Input: part model. Units: mm. Frame: model coordinates. Face numbers are marked on the shaded views. A direction names the side the tool comes from. Give positions to 0.01 mm unless a question says otherwise; leave off trailing zeros. Write each loop counter-clockwise with the first axis right and the second up, starting at its lowest first coordinate (ties: lowest second). Pieces come first, ordered by that corner, then holes. Notation, with made-up numbers: (-34.5, -1.75) - (-11.5, -1.75) arc R33 cw to (-11.5, 27.25) - close; hole circle Ø4 at (-27.75, 49.5). An arc over 180 degrees is marked (long way). Use a Markdown table: item, result. Add a question column.
1. Set-up query: the marked faces 1 and 2. Return all of +Z, -Z, +X, -X, +Y, -Y with unobstructed straight access to the full face (end or side cutting, diameter ignored); none if empty.
2. Section query C-C, the plane z = -82. Return loops of the section in (x, y).
3. Material intervals for probe 1 along Z at (x, y) = (-10.5, -1.5); probe 2 along X at (y, z) = (25, -56.5); probe 3 along Y at (x, z) = (-47, -80), sorted ascending.
4. Section query A-A, the plane y = 0. Count the separate pieces of the cut face and the enclosed holes in it, plus the area to 3 significant figures.
5. Pin query (flat end, axial travel): pin 1 (1.5 mm diameter, centred on x = -14.5, z = -94, fed in from -Y); pin 2 (4 mm diameter, centred on x = 39, y = 44.5, fed in from -Z); pin 3 (2 mm diameter, centred on y = -45, z = -132, fed in from +X); pin 4 (12 mm diameter, centred on x = 35, y = 0, fed in from +Z). Return the tip coordinate at first contact, or that it passes through.
```python
from build123d import *

# Parameters (mm, degrees)
F0_R     = 75
F0_R_2   = 10
F1_DEPTH = 5
F2_R     = 4.99999
F3_R     = 7.5
F4_DEPTH = 150


# Not quite as in the source:
# - a fillet or chamfer is up to 0.001 mm smaller than in the source, because OpenCascade refuses the exact size


with BuildPart() as f1:
    # F0 (on Top) → F1 (new body)
    with BuildSketch(Plane.XY):
        Circle(F0_R)
        with Locations((-24.7487373415, -24.7487373415)):
            Circle(F0_R_2, mode=Mode.SUBTRACT)
        with Locations((0, -35)):
            Circle(F0_R_2, mode=Mode.SUBTRACT)
        with Locations((24.7487373415, -24.7487373415)):
            Circle(F0_R_2, mode=Mode.SUBTRACT)
        with Locations((-35, 0)):
            Circle(F0_R_2, mode=Mode.SUBTRACT)
        with Locations((-24.7487373415, 24.7487373415)):
            Circle(F0_R_2, mode=Mode.SUBTRACT)
        with Locations((35, 0)):
            Circle(F0_R_2, mode=Mode.SUBTRACT)
        with Locations((0, 35)):
            Circle(F0_R_2, mode=Mode.SUBTRACT)
        with Locations((24.7487373415, 24.7487373415)):
            Circle(F0_R_2, mode=Mode.SUBTRACT)
    extrude(amount=F1_DEPTH)

    # F2 (radius 5 in the source; OpenCascade refuses exactly that, so slightly less here)
    f2_edges = [f1.edges().sort_by_distance(p)[0] for p in [
        (-75, 0, 5),
    ]]
    fillet(f2_edges, radius=F2_R)

    # F3 (on face) → F4 (join)
    with BuildSketch(Plane.XY):
        with Locations((21.2406198754, 50.7329879596)):
            Circle(F3_R)
        with Locations((-50.7329879596, 21.2406198754)):
            Circle(F3_R)
        with Locations((-21.2406198754, -50.7329879596)):
            Circle(F3_R)
        with Locations((50.7329879596, -21.2406198754)):
            Circle(F3_R)
    extrude(amount=-F4_DEPTH)


solid = f1.part
```
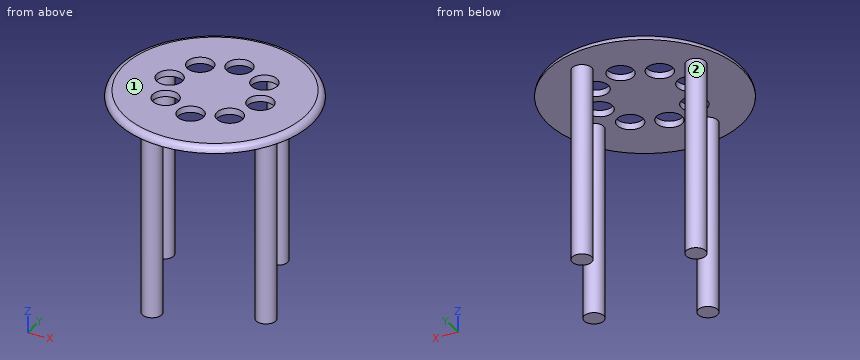
Result sheet:
| question | item | result |
|---|---|---|
| 1 | face 1 | +Z, +X, -X, +Y, -Y |
| 1 | face 2 | -Z |
| 2 | outline | circle Ø15 at (-50.73, 21.24); circle Ø15 at (-21.24, -50.73); circle Ø15 at (21.24, 50.73); circle Ø15 at (50.73, -21.24) |
| 3 | probe 1 | z = 0 to 5 |
| 3 | probe 2 | x = -57.22 to -44.24 |
| 3 | probe 3 | y = 14.74 to 27.75 |
| 4 | separate pieces | 3 |
| 4 | enclosed holes | 0 |
| 4 | area | 539 mm² |
| 5 | pin 1 | stops at y = -55.25 |
| 5 | pin 2 | stops at z = 0 |
| 5 | pin 3 | stops at x = -15.42 |
| 5 | pin 4 | passes through |
